The model under review builds one solid part; all positions refer to its coordinate system, in mm. A direction names the side the tool comes from. Coordinates: 2 decimals unless noted, no trailing zeros. Write each loop counter-clockwise with the first axis right and the second up, starting at its lowest first coordinate (ties: lowest second). Pieces come first, ordered by that corner, then holes. Notation, with made-up numbers: (11, 60) -> (49, 60) arc R17 cw to (49, 90) -> close; hole circle Ø7 at (-1, 87.25). An arc over 180 degrees is marked (long way). Write each question's results on one line, items separated by ' | '.
```python
from build123d import *

# Parameters (mm, degrees)
EXTRUDE_1_DEPTH     = 5
SKETCH_2_3_R        = 1.5
CUT_EXTRUDE_1_DEPTH = 5
SKETCH_3_R          = 1.5
CUT_EXTRUDE_2_DEPTH = 10
SKETCH_4_R          = 1.5
CUT_EXTRUDE_3_DEPTH = 33


with BuildPart() as part:
    # Sketch 2 → Extrude 1 (new body)
    with BuildSketch(Plane.XY):
        with BuildLine():
            Line((2769.066394733, 1854.135920645), (2815.285788336, 1854.135920645))
            ThreePointArc((2815.285788336, 1854.135920645), (2822.615812871, 1855.527569285), (2828.925755538, 1859.508846613))
            Line((2828.925755538, 1859.508846613), (2883.306876366, 1910.220062186))
            ThreePointArc((2883.306876366, 1910.220062186), (2886.89136565, 1911.560247813), (2890.373636674, 1909.973285478))
            Line((2890.373636674, 1909.973285478), (2910.833587476, 1888.03267443))
            ThreePointArc((2910.833587476, 1888.03267443), (2912.173773103, 1884.448185146), (2910.586810768, 1880.965914121))
            Line((2910.586810768, 1880.965914121), (2863.536124333, 1837.090439207))
            ThreePointArc((2863.536124333, 1837.090439207), (2858.834890047, 1830.438346554), (2857.176091534, 1822.463365175))
            Line((2857.176091534, 1822.463365175), (2857.176091534, 1745.808476115))
            ThreePointArc((2857.176091534, 1745.808476115), (2858.834890047, 1737.833494737), (2863.536124333, 1731.181402083))
            Line((2863.536124333, 1731.181402083), (2910.586810768, 1687.305927169))
            ThreePointArc((2910.586810768, 1687.305927169), (2912.173773103, 1683.823656144), (2910.833587476, 1680.239166861))
            Line((2910.833587476, 1680.239166861), (2890.373636674, 1658.298555812))
            ThreePointArc((2890.373636674, 1658.298555812), (2886.89136565, 1656.711593477), (2883.306876366, 1658.051779104))
            Line((2883.306876366, 1658.051779104), (2828.925755538, 1708.762994677))
            ThreePointArc((2828.925755538, 1708.762994677), (2822.615812871, 1712.744272005), (2815.285788336, 1714.135920645))
            Line((2815.285788336, 1714.135920645), (2769.066394733, 1714.135920645))
            ThreePointArc((2769.066394733, 1714.135920645), (2761.736370198, 1712.744272005), (2755.426427531, 1708.762994677))
            Line((2755.426427531, 1708.762994677), (2701.045306703, 1658.051779104))
            ThreePointArc((2701.045306703, 1658.051779104), (2697.460817419, 1656.711593477), (2693.978546395, 1658.298555812))
            Line((2693.978546395, 1658.298555812), (2673.518595593, 1680.239166861))
            ThreePointArc((2673.518595593, 1680.239166861), (2672.178409966, 1683.823656144), (2673.765372301, 1687.305927169))
            Line((2673.765372301, 1687.305927169), (2720.816058736, 1731.181402083))
            ThreePointArc((2720.816058736, 1731.181402083), (2725.517293022, 1737.833494737), (2727.176091534, 1745.808476115))
            Line((2727.176091534, 1745.808476115), (2727.176091534, 1822.463365175))
            ThreePointArc((2727.176091534, 1822.463365175), (2725.517293022, 1830.438346554), (2720.816058736, 1837.090439207))
            Line((2720.816058736, 1837.090439207), (2673.765372301, 1880.965914121))
            ThreePointArc((2673.765372301, 1880.965914121), (2672.178409966, 1884.448185146), (2673.518595593, 1888.03267443))
            Line((2673.518595593, 1888.03267443), (2693.978546395, 1909.973285478))
            ThreePointArc((2693.978546395, 1909.973285478), (2697.460817419, 1911.560247813), (2701.045306703, 1910.220062186))
            Line((2701.045306703, 1910.220062186), (2755.426427531, 1859.508846613))
            ThreePointArc((2755.426427531, 1859.508846613), (2761.736370198, 1855.527569285), (2769.066394733, 1854.135920645))
        make_face()
    extrude(amount=EXTRUDE_1_DEPTH)

    # Sketch 2_3 → Cut-Extrude 1 (cut)
    with BuildSketch(Plane.XY):
        with Locations((2899.625481666, 1891.254221285)):
            Circle(SKETCH_2_3_R)
        with Locations((2892.805498065, 1898.567758302)):
            Circle(SKETCH_2_3_R)
        with Locations((2857.700520387, 1865.831837019)):
            Circle(SKETCH_2_3_R)
        with Locations((2864.520503988, 1858.518300002)):
            Circle(SKETCH_2_3_R)
        with Locations((2892.805498065, 1669.704082989)):
            Circle(SKETCH_2_3_R)
        with Locations((2864.520503988, 1709.753541288)):
            Circle(SKETCH_2_3_R)
        with Locations((2857.700520387, 1702.440004272)):
            Circle(SKETCH_2_3_R)
        Polygon((2697.882091611, 1668.775307921), (2684.242124409, 1683.402381953), (2713.496272474, 1710.682316356), (2727.136239676, 1696.055242323), align=None)
        Polygon((2886.470091458, 1668.775307921), (2857.215943393, 1696.055242323), (2870.855910595, 1710.682316356), (2900.110058659, 1683.402381953), align=None)
        Polygon((2697.882091611, 1899.496533369), (2727.136239676, 1872.216598967), (2713.496272474, 1857.589524935), (2684.242124409, 1884.869459337), align=None)
        with Locations((2691.546685004, 1898.567758302)):
            Circle(SKETCH_2_3_R)
        Polygon((2870.855910595, 1857.589524935), (2900.110058659, 1884.869459337), (2886.470091458, 1899.496533369), (2857.215943393, 1872.216598967), align=None)
        with Locations((2899.625481666, 1677.017620005)):
            Circle(SKETCH_2_3_R)
        with Locations((2726.651662682, 1702.440004272)):
            Circle(SKETCH_2_3_R)
        with Locations((2719.831679081, 1709.753541288)):
            Circle(SKETCH_2_3_R)
        with Locations((2691.546685004, 1669.704082989)):
            Circle(SKETCH_2_3_R)
        with Locations((2684.726701403, 1677.017620005)):
            Circle(SKETCH_2_3_R)
        with Locations((2726.651662682, 1865.831837019)):
            Circle(SKETCH_2_3_R)
        with Locations((2719.831679081, 1858.518300002)):
            Circle(SKETCH_2_3_R)
        with Locations((2684.726701403, 1891.254221285)):
            Circle(SKETCH_2_3_R)
    extrude(amount=CUT_EXTRUDE_1_DEPTH, mode=Mode.SUBTRACT)

    # Sketch 3 → Cut-Extrude 2 (cut)
    with BuildSketch(Plane(origin=(0, 0, 0), x_dir=(-1, 0, 0), z_dir=(0, 0, -1))):
        with Locations((-2888.892976427, 1700.699117662)):
            Circle(SKETCH_3_R)
        with Locations((-2868.433025626, 1678.758506614)):
            Circle(SKETCH_3_R)
        with Locations(Location((-2715.919157443, 1678.758506614, 0), (0, 0, 180))):
            Circle(SKETCH_3_R)
        with Locations(Location((-2695.459206642, 1700.699117662, 0), (0, 0, 180))):
            Circle(SKETCH_3_R)
        with Locations((-2695.459206642, 1867.572723628)):
            Circle(SKETCH_3_R)
        with Locations((-2715.919157443, 1889.513334676)):
            Circle(SKETCH_3_R)
        with Locations(Location((-2868.433025626, 1889.513334676, 0), (0, 0, 180))):
            Circle(SKETCH_3_R)
        with Locations(Location((-2888.892976427, 1867.572723628, 0), (0, 0, 180))):
            Circle(SKETCH_3_R)
    extrude(amount=-CUT_EXTRUDE_2_DEPTH, mode=Mode.SUBTRACT)

    # Sketch 4 → Cut-Extrude 3 (cut)
    with BuildSketch(Plane(origin=(0, 0, 0), x_dir=(-1, 0, 0), z_dir=(0, 0, -1))):
        with Locations((-2865.391879185, 1722.614245382)):
            Circle(SKETCH_4_R)
        with Locations((-2855.161903784, 1711.643939858)):
            Circle(SKETCH_4_R)
        with Locations(Location((-2844.931928383, 1700.673634334, 0), (0, 0, 180))):
            Circle(SKETCH_4_R)
        with Locations((-2739.420254686, 1700.673634334)):
            Circle(SKETCH_4_R)
        with Locations(Location((-2729.190279285, 1711.643939858, 0), (0, 0, 180))):
            Circle(SKETCH_4_R)
        with Locations(Location((-2718.960303884, 1722.614245382, 0), (0, 0, 180))):
            Circle(SKETCH_4_R)
        with Locations((-2718.960303884, 1845.657595908)):
            Circle(SKETCH_4_R)
        with Locations((-2729.190279285, 1856.627901432)):
            Circle(SKETCH_4_R)
        with Locations(Location((-2739.420254686, 1867.598206957, 0), (0, 0, 180))):
            Circle(SKETCH_4_R)
        with Locations((-2844.931928383, 1867.598206957)):
            Circle(SKETCH_4_R)
        with Locations(Location((-2855.161903784, 1856.627901432, 0), (0, 0, 180))):
            Circle(SKETCH_4_R)
        with Locations(Location((-2865.391879185, 1845.657595908, 0), (0, 0, 180))):
            Circle(SKETCH_4_R)
    extrude(amount=-CUT_EXTRUDE_3_DEPTH, mode=Mode.SUBTRACT)


solid = part.part
```
Q1. Clearance check with flat-ended pins moving along their axes: P1, Ø2.5, axis at x = 2864.52, y = 1709.75, coming from the -Z side; P2, Ø1, axis at x = 2726.5, z = 3, coming from the -Y side. State where each tip first meets the part, or that it passes through.
Solution:
P1: through | P2: y = 1681.32
Q2. Add section B-B (x = 2709). Write out the cut boundary in (y, z), plus the area to 3 significant figures.
Solution:
outline: (1665.47, 0) -> (1679.14, 0) -> (1679.14, 5) -> (1665.47, 5) -> close; (1706.49, 0) -> (1720.16, 0) -> (1720.16, 5) -> (1706.49, 5) -> close; (1848.11, 0) -> (1861.78, 0) -> (1861.78, 5) -> (1848.11, 5) -> close; (1889.13, 0) -> (1902.8, 0) -> (1902.8, 5) -> (1889.13, 5) -> close | area: 273 mm²
Q3. Machinability: for faces 5 (the flat face through (2696.961, 1708.937, 2.465)), 6 (the flat face through (2872.05, 1682.22, 2.46)), 7 (the flat face through (2728.617, 1683.762, 2.465)), 8 (the flat face through (2855.736, 1884.509, 2.465)), which of the approach directions +Z, -Z, +X, -X, +Y, -Y give a long, thin tool a straight path to every point of the face, cutting with its end or side? Answer none if there is none.
Solution:
face 5: +Z, -Z, -X | face 6: +Z, -Z | face 7: +Z, -Z, -Y | face 8: +Z, -Z, +Y
Q4. Add section A-A (y = 1876). Write out the cut boundary in (x, z).
Solution:
outline: (2679.09, 0) -> (2693.75, 0) -> (2693.75, 5) -> (2679.09, 5) -> close; (2723.08, 0) -> (2737.74, 0) -> (2737.74, 5) -> (2723.08, 5) -> close; (2846.61, 0) -> (2861.27, 0) -> (2861.27, 5) -> (2846.61, 5) -> close; (2890.6, 0) -> (2905.26, 0) -> (2905.26, 5) -> (2890.6, 5) -> close
Q5. Add section C-C (y = 1796.5). Write out the cut boundary in (x, z), plus the area to 3 significant figures.
Solution:
outline: (2727.18, 0) -> (2857.18, 0) -> (2857.18, 5) -> (2727.18, 5) -> close | area: 650 mm²
Q6. Draft analysis for pull direction X (two halves, no side actions). For faces 1 (the flat face through (2794, 1786, 5)), 2 (the flat face through (2691.158, 1675.986, 2.465)), 3 (the flat face through (2697.62, 1858.72, 2.46)), 4 (the cylindrical face through (2858.88, 1830.54, 2.46)), state which applies: pulls with the +X half, pulls with the -X half, needs draft (parallel to the pull), parting line crosses it, or undercut.
Solution:
face 1: needs draft | face 2: undercut | face 3: pulls with the -X half | face 4: pulls with the +X half
Q7. Add section D-D (x = 2749). Write out the cut boundary in (y, z).
Solution:
outline: (1702.77, 0) -> (1865.5, 0) -> (1865.5, 5) -> (1702.77, 5) -> close
Q8. For line 1 (X direction, y = 1871, z = 1.55); line 2 (X direction, y = 1888.5, z = 0.2); line 3 (Y direction, x = 2871, z = 1.6), list the stretches that pass through material, from the lowest coordinate up. Write a range as from..to.
Solution:
line 1: 2684.45..2699.12, 2726..2743.1, 2841.25..2858.35, 2885.24..2899.9 | line 2: 2673.95..2687.63, 2709.67..2714.81, 2717.03..2724.34, 2860.01..2867.33, 2869.54..2874.68, 2896.72..2910.4 | line 3: 1669.53..1683.2, 1710.55..1724.22, 1844.05..1857.72, 1885.07..1898.74
